```python
from build123d import *

# Parameters (mm, degrees)
F1_DEPTH = 1342.9996
F3_DEPTH = 63.4248


with BuildPart() as f1:
    # F0 (on Right) → F1 (new body)
    with BuildSketch(Plane.YZ):
        with BuildLine():
            Line((76.2, 0), (-76.2, 0))
            Line((-76.2, 0), (-76.2, -63.4238))
            ThreePointArc((-76.2, -63.4238), (-72.574321, -62.102069), (-70.649887, -58.757061))
            Line((-70.649887, -58.757061), (-63.124886, -15.566335))
            ThreePointArc((-63.124886, -15.566335), (-59.952782, -10.052651), (-53.976459, -7.874))
            Line((-53.976459, -7.874), (53.976459, -7.874))
            ThreePointArc((53.976459, -7.874), (59.952782, -10.052651), (63.124886, -15.566335))
            Line((63.124886, -15.566335), (70.649887, -58.757061))
            ThreePointArc((70.649887, -58.757061), (72.574321, -62.102069), (76.2, -63.4238))
            Line((76.2, -63.4238), (76.2, 0))
        make_face()
    extrude(amount=F1_DEPTH)

    # F2 (on face) → F3 (cut, through all)
    with BuildSketch(Plane.XY):
        with BuildLine():
            Line((1342.9996, -76.2), (1342.9996, 76.2))
            Line((1342.9996, 76.2), (1279.5758, 76.2))
            ThreePointArc((1279.5758, 76.2), (1280.897531, 72.574321), (1284.242539, 70.649887))
            Line((1284.242539, 70.649887), (1327.433265, 63.124886))
            ThreePointArc((1327.433265, 63.124886), (1332.946949, 59.952782), (1335.1256, 53.976459))
            Line((1335.1256, 53.976459), (1335.1256, -53.976459))
            ThreePointArc((1335.1256, -53.976459), (1332.946949, -59.952782), (1327.433265, -63.124886))
            Line((1327.433265, -63.124886), (1284.242539, -70.649887))
            ThreePointArc((1284.242539, -70.649887), (1280.897531, -72.574321), (1279.5758, -76.2))
            Line((1279.5758, -76.2), (1342.9996, -76.2))
        make_face()
        with BuildLine():
            Line((7.874, -53.976459), (7.874, 53.976459))
            ThreePointArc((7.874, 53.976459), (10.052651, 59.952782), (15.566335, 63.124886))
            Line((15.566335, 63.124886), (58.757061, 70.649887))
            ThreePointArc((58.757061, 70.649887), (62.102069, 72.574321), (63.4238, 76.2))
            Line((63.4238, 76.2), (0, 76.2))
            Line((0, 76.2), (0, -76.2))
            Line((0, -76.2), (63.4238, -76.2))
            ThreePointArc((63.4238, -76.2), (62.102069, -72.574321), (58.757061, -70.649887))
            Line((58.757061, -70.649887), (15.566335, -63.124886))
            ThreePointArc((15.566335, -63.124886), (10.052651, -59.952782), (7.874, -53.976459))
        make_face()
    extrude(amount=-F3_DEPTH, mode=Mode.SUBTRACT)


solid = f1.part
```
Verification items for the finished model (mm, model axes). A direction names the side the tool comes from. Round coordinates to 2 decimals unless told otherwise and drop trailing zeros. Write each loop counter-clockwise with the first axis right and the second up, starting at its lowest first coordinate (ties: lowest second). Pieces come first, ordered by that corner, then holes. Notation, with made-up numbers: (62.25, -23) - (112.25, -23) arc R26 ccw to (112.25, -6) - close; hole circle Ø7 at (-23, -30). An arc over 180 degrees is marked (long way). Answer as a JSON object with one key per item and string values. Group by question number.
Q1. Section check C-C, the plane y = 23. Enter the section's corners in (x, z), plus the area to 3 significant figures.
Q2. Tool access check on faces 4 (the flat face through (663, 76.2, -32)), 5 (the flat face through (662.32, -66.94, -37.46)). Record the directions out of +Z, -Z, +X, -X, +Y, -Y that give a thin tool (end or side, any length) a straight path to the whole face; none if there is none.
Q3. Section check A-A, the plane z = -45. Enter the section's corners in (x, y), plus the area to 3 significant figures.
Q4. Thickness scan on line 1 (Y direction, x = 1065, z = -17.5); line 2 (Z direction, x = 747.5, y = -29); line 3 (Y direction, x = 811.5, z = -57). Record the ranges inside material, lowest first.
Q5. Section check B-B, the plane x = 88.5. Enter the section's corners in (y, z).
Q6. Mould release check, pull along Y, two halves, no side actions. Record for faces 1 (the flat face through (662.317, 66.835, -36.859)), 2 (the flat face through (41.66, 67.67, -22.44)), 3 (the flat face through (662, 1, 0)): released by +Y, released by -Y, zero draft, split by the parting line, or undercut.
Found:
{
 "1": {"outline": "(7.87, -7.87) - (1335.13, -7.87) - (1335.13, 0) - (7.87, 0) - close", "area": "10,500 mm^2"},
 "2": {"face 4": "+Z, -Z, +X, -X, +Y", "face 5": "-Z, +X, -X"},
 "3": {"outline": "(45, -68.25) - (58.76, -70.65) arc R5.63 cw to (63.42, -76.2) - (1279.58, -76.2) arc R5.63 cw to (1284.24, -70.65) - (1298, -68.25) - close; (45, 68.25) - (1298, 68.25) - (1284.24, 70.65) arc R5.63 cw to (1279.58, 76.2) - (63.42, 76.2) arc R5.63 cw to (58.76, 70.65) - close", "area": "19,500 mm^2"},
 "4": {"line 1": "y = -76.2 to -63.46, 63.46 to 76.2", "line 2": "z = -7.87 to 0", "line 3": "y = -76.2 to -70.34, 70.34 to 76.2"},
 "5": {"outline": "(-76.2, -63.42) arc R5.63 ccw to (-70.65, -58.76) - (-63.12, -15.57) arc R9.29 cw to (-53.98, -7.87) - (53.98, -7.87) arc R9.29 cw to (63.12, -15.57) - (70.65, -58.76) arc R5.63 ccw to (76.2, -63.42) - (76.2, 0) - (-76.2, 0) - close"},
 "6": {"face 1": "undercut", "face 2": "released by +Y", "face 3": "zero draft"}
}
